Could you check a few things on this drawing? It's one solid part, dimensions in mm from its lowest x, y, z. A direction names the side the tool comes from. Round coordinates to 2 decimals unless told otherwise and drop trailing zeros. Write each loop counter-clockwise with the first axis right and the second up, starting at its lowest first coordinate (ties: lowest second). Pieces come first, ordered by that corner, then holes. Notation, with made-up numbers: (44, 8) -> (59, 8) arc R9 ccw to (59, 19) -> close; hole circle Ø3 at (78, -14). An arc over 180 degrees is marked (long way). Answer in a Markdown table with one row per item.
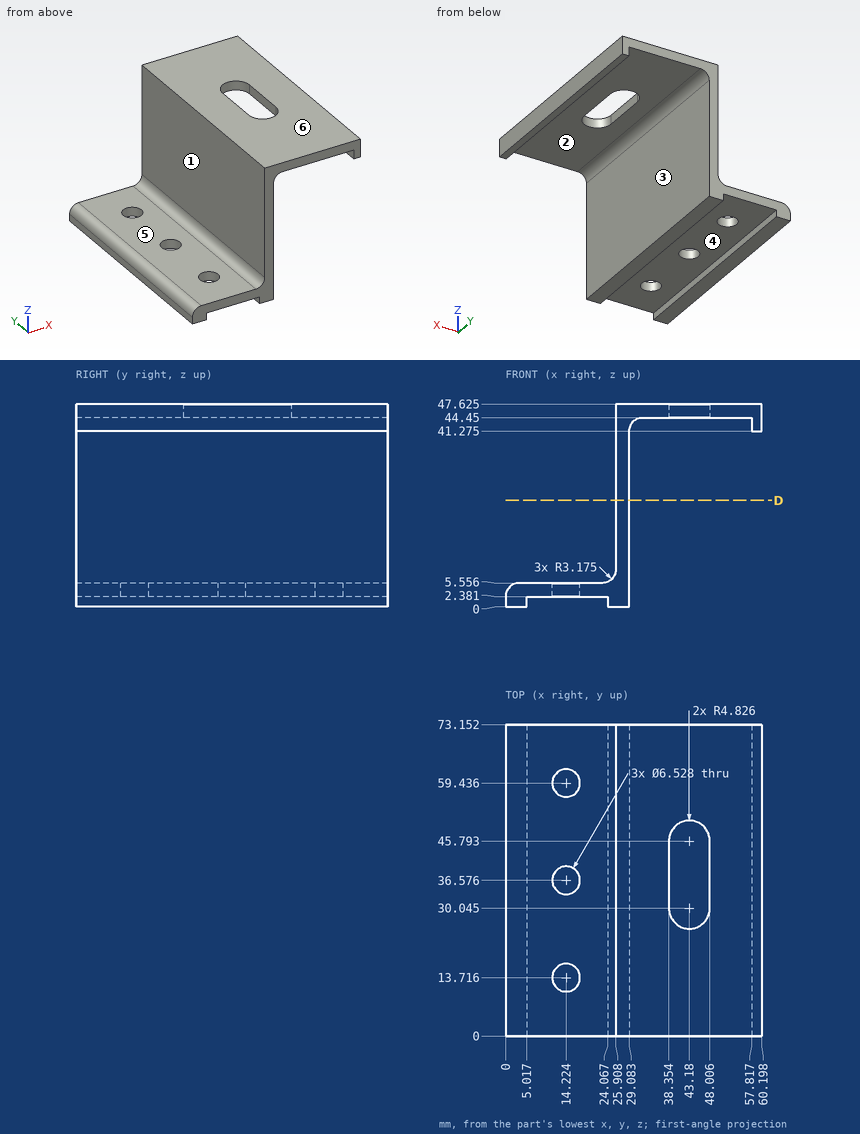
1) I need wall thicknesses on line 1 (X direction, y = 43, z = 21.5); line 2 (Z direction, x = 19, y = 68); line 3 (X direction, y = 12, z = 46.5). Which ranges of each line are inside material? Lowest first, please. Write a range as [from, to].
Response:
| item | result |
|---|---|
| line 1 | x = [25.91, 29.08] |
| line 2 | z = [2.38, 5.56] |
| line 3 | x = [25.91, 60.2] |
2) We'd pull the mould along X, two halves only. Please class the marked faces 1, 2, 3 and 4: +X half, -X half, draft (parallel to the pull), parting line (faces both ways), or undercut.
Response:
| item | result |
|---|---|
| face 1 | -X half |
| face 2 | undercut |
| face 3 | +X half |
| face 4 | undercut |
3) For pin 1 (1.9 mm diameter, centred on x = 59.5, y = 19, fed in from -Z) (1 decimal); pin 2 (7.5 mm diameter, centred on x = 41.5, y = 24.5, fed in from -Z); pin 3 (19.5 mm diameter, centred on y = 32, z = 28, fed in from -X); pin 4 (21 mm diameter, centred on x = 17.5, y = 54, fed in from -Z), each with a flat end and sliding along its axis, tell me the tip position at first contact or that it passes through.
Response:
| item | result |
|---|---|
| pin 1 | stops at z = 41.3 |
| pin 2 | stops at z = 44.45 |
| pin 3 | stops at x = 25.91 |
| pin 4 | stops at z = 0 |
4) I want a section at D-D, the plane z = 25. List the corners of the cut face in (x, y) for me, and give its area (3 significant figures).
Response:
| item | result |
|---|---|
| outline | (25.91, 0) -> (29.08, 0) -> (29.08, 73.15) -> (25.91, 73.15) -> close |
| area | 232 mm^2 |
5) Which directions (+Z, -Z, +X, -X, +Y, -Y) give clear straight access to the entire face, cutting with the end or side of a thin tool? Please do the marked faces 5 and 6.
Response:
| item | result |
|---|---|
| face 5 | +Z, -X, +Y, -Y |
| face 6 | +Z, +X, -X, +Y, -Y |
